Read the model definition and answer for the solid it produces. Units are mm, in the model's axes. Round coordinates to 2 decimals unless told otherwise and drop trailing zeros. Write each loop counter-clockwise with the first axis right and the second up, starting at its lowest first coordinate (ties: lowest second). Pieces come first, ordered by that corner, then holes.
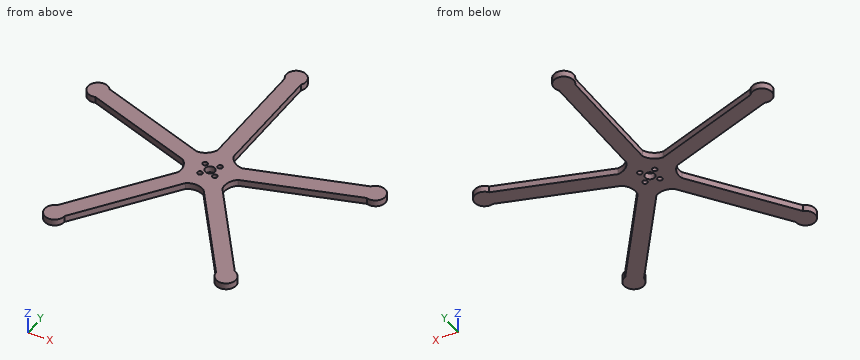
from build123d import *

# Parameters (mm, degrees)
F0_R     = 1.905
F0_R_2   = 3.81
F1_DEPTH = 5.08


with BuildPart() as f1:
    # F0 (on Top) → F1 (new body)
    with BuildSketch(Plane.XY):
        with BuildLine():
            ThreePointArc((-6.35, 24.901362), (-10.804149, 19.10083), (-17.697191, 16.657146))
            Line((-17.697191, 16.657146), (-102.246115, 44.128757))
            ThreePointArc((-102.246115, 44.128757), (-115.956738, 41.906823), (-106.170631, 32.050339))
            Line((-106.170631, 32.050339), (-21.621706, 4.578728))
            ThreePointArc((-21.621706, 4.578728), (-17.48148, -1.449882), (-17.287465, -8.760695))
            Line((-17.287465, -8.760695), (-69.541574, -80.682305))
            ThreePointArc((-69.541574, -80.682305), (-71.665205, -94.408498), (-59.267058, -88.147178))
            Line((-59.267058, -88.147178), (-7.01295, -16.225567))
            ThreePointArc((-7.01295, -16.225567), (0, -14.150921), (7.01295, -16.225567))
            Line((7.01295, -16.225567), (59.267058, -88.147178))
            ThreePointArc((59.267058, -88.147178), (71.665205, -94.408498), (69.541574, -80.682305))
            Line((69.541574, -80.682305), (17.287465, -8.760695))
            ThreePointArc((17.287465, -8.760695), (17.48148, -1.449882), (21.621706, 4.578728))
            Line((21.621706, 4.578728), (106.170631, 32.050339))
            ThreePointArc((106.170631, 32.050339), (115.956738, 41.906823), (102.246115, 44.128757))
            Line((102.246115, 44.128757), (17.697191, 16.657146))
            ThreePointArc((17.697191, 16.657146), (10.804149, 19.10083), (6.35, 24.901362))
            Line((6.35, 24.901362), (6.35, 113.801362))
            ThreePointArc((6.35, 113.801362), (0, 126.154324), (-6.35, 113.801362))
            Line((-6.35, 113.801362), (-6.35, 24.901362))
        make_face()
        with Locations((-4.141972, -2.013932)):
            Circle(F0_R, mode=Mode.SUBTRACT)
        with Locations((0, 4.230195)):
            Circle(F0_R_2, mode=Mode.SUBTRACT)
        with Locations((-6.244127, 8.372167)):
            Circle(F0_R, mode=Mode.SUBTRACT)
        with Locations((6.244127, 0.088223)):
            Circle(F0_R, mode=Mode.SUBTRACT)
        with Locations((4.141972, 10.474322)):
            Circle(F0_R, mode=Mode.SUBTRACT)
    extrude(amount=F1_DEPTH)


solid = f1.part
Q1. Section A-A (x = -35) is taken. Determine the outline of the cut face in (y, z).
Verdict:
outline: (-54.75, 0) - (-33.14, 0) - (-33.14, 5.08) - (-54.75, 5.08) - close; (8.93, 0) - (22.28, 0) - (22.28, 5.08) - (8.93, 5.08) - close
Q2. Section D-D (y = 63) is taken. Determine the outline of the cut face in (x, z), then the cut area to 3 significant figures.
Verdict:
outline: (-6.35, 0) - (6.35, 0) - (6.35, 5.08) - (-6.35, 5.08) - close
area: 64.5 mm2
Q3. Straight lines are drawn through the part: probe 1 along X at (y, z) = (-65.5, 0.3); probe 2 along X at (y, z) = (58.5, 4.6); probe 3 along X at (y, z) = (-28, 4.55). For each, find the intervals that lie inside material, in ascending order.
Verdict:
probe 1: x = -58.51 to -42.81, 42.81 to 58.51
probe 2: x = -6.35 to 6.35
probe 3: x = -31.27 to -15.57, 15.57 to 31.27
Q4. Section C-C (z = 2.3) is taken. Determine the outline of the cut face in (x, y) (3 decimals), then the cut area to 3 significant figures.
Verdict:
outline: (-106.171, 32.05) - (-21.622, 4.579) arc R12.89 cw to (-17.287, -8.761) - (-69.542, -80.682) arc R7.809 ccw (long way) to (-59.267, -88.147) - (-7.013, -16.226) arc R12.89 cw to (7.013, -16.226) - (59.267, -88.147) arc R7.809 ccw (long way) to (69.542, -80.682) - (17.287, -8.761) arc R12.89 cw to (21.622, 4.579) - (106.171, 32.05) arc R7.809 ccw (long way) to (102.246, 44.129) - (17.697, 16.657) arc R12.89 cw to (6.35, 24.901) - (6.35, 113.801) arc R7.809 ccw (long way) to (-6.35, 113.801) - (-6.35, 24.901) arc R12.89 cw to (-17.697, 16.657) - (-102.246, 44.129) arc R7.809 ccw (long way) to start; hole circle Ø3.81 at (-6.244, 8.372); hole circle Ø3.81 at (-4.142, -2.014); hole circle Ø7.62 at (0, 4.23); hole circle Ø3.81 at (4.142, 10.474); hole circle Ø3.81 at (6.244, 0.088)
area: 7,640 mm2
Q5. Section B-B (y = -66.5) is taken. Determine the outline of the cut face in (x, z).
Verdict:
outline: (-59.24, 0) - (-43.54, 0) - (-43.54, 5.08) - (-59.24, 5.08) - close; (43.54, 0) - (59.24, 0) - (59.24, 5.08) - (43.54, 5.08) - close
Q6. Flat-ended cylindrical pins translate along their axes: pin 1 Ø3.5 at (x, y) = (-6.24, 8.37) entering from +Z; pin 2 Ø1 at (x, z) = (-14.5, 1.5) entering from -Y; pin 3 Ø3 at (x, z) = (-37.5, 3.5) entering from -Y. Find the tip coordinate at first contact, or state that the pin passes through.
Verdict:
pin 1: passes through
pin 2: stops at y = -27.22
pin 3: stops at y = -60.25
